The model under review builds one solid part; all positions refer to its coordinate system, in mm. A direction names the side the tool comes from. Round coordinates to 2 decimals unless told otherwise and drop trailing zeros. Write each loop counter-clockwise with the first axis right and the second up, starting at its lowest first coordinate (ties: lowest second). Pieces come first, ordered by that corner, then holes. Notation, with made-up numbers: (-38.75, 66.25) - (-31.75, 66.25) arc R27 cw to (-31.75, 87.25) - close; hole circle Ø1 at (11, 21). An arc over 180 degrees is marked (long way). Return JSON: item names as keys, results as strings.
from build123d import *

# Parameters (mm, degrees)
SKETCH_1_R          = 1.6
SKETCH_1_W          = 11.667697598
SKETCH_1_H          = 6.517356375
SKETCH_1_W_2        = 22
SKETCH_1_H_2        = 5
EXTRUDE_1_DEPTH     = 3
SKETCH_2_W          = 75.93825213
SKETCH_2_H          = 5.545458332
EXTRUDE_2_DEPTH     = 8
SKETCH_3_R          = 1.8
CUT_EXTRUDE_1_DEPTH = 15


with BuildPart() as part:
    # 草图1 → 凸台-拉伸1 (new body)
    with BuildSketch(Plane(origin=(0, 0, 0), x_dir=(1, 0, 0), z_dir=(0, 1, 0))):
        with BuildLine():
            Line((-49.5, -40), (49.5, -40))
            ThreePointArc((49.5, -40), (50.914213562, -39.414213562), (51.5, -38))
            Line((51.5, -38), (51.5, 38))
            ThreePointArc((51.5, 38), (50.914213562, 39.414213562), (49.5, 40))
            Line((49.5, 40), (20.187430173, 40))
            Line((20.187430173, 40), (20.187430173, 26.249140852))
            Line((20.187430173, 26.249140852), (-20.187430173, 26.249140852))
            Line((-20.187430173, 26.249140852), (-20.187430173, 40))
            Line((-20.187430173, 40), (-49.5, 40))
            ThreePointArc((-49.5, 40), (-50.914213562, 39.414213562), (-51.5, 38))
            Line((-51.5, 38), (-51.5, -38))
            ThreePointArc((-51.5, -38), (-50.914213562, -39.414213562), (-49.5, -40))
        make_face()
        with Locations(Location((-43.3, -31.8, 0), (0, 0, 270))):
            Circle(SKETCH_1_R, mode=Mode.SUBTRACT)
        with Locations((-30.135277266, -31.195863481)):
            Rectangle(SKETCH_1_W, SKETCH_1_H, mode=Mode.SUBTRACT)
        with Locations(Location((-42.391806281, -12.03, 0), (0, 0, 270))):
            Circle(SKETCH_1_R, mode=Mode.SUBTRACT)
        with Locations(Location((-33.901806281, -12.03, 0), (0, 0, 270))):
            Circle(SKETCH_1_R, mode=Mode.SUBTRACT)
        with Locations((0, -31.19586348)):
            Rectangle(SKETCH_1_W_2, SKETCH_1_H_2, mode=Mode.SUBTRACT)
        with Locations((30.135277266, -31.195863481)):
            Rectangle(SKETCH_1_W, SKETCH_1_H, mode=Mode.SUBTRACT)
        with Locations(Location((43.3, -31.8, 0), (0, 0, 270))):
            Circle(SKETCH_1_R, mode=Mode.SUBTRACT)
        with Locations(Location((33.901806281, -12.03, 0), (0, 0, 270))):
            Circle(SKETCH_1_R, mode=Mode.SUBTRACT)
        with Locations(Location((42.391806281, -12.03, 0), (0, 0, 270))):
            Circle(SKETCH_1_R, mode=Mode.SUBTRACT)
        with Locations(Location((-42.391806281, 12.03, 0), (0, 0, 270))):
            Circle(SKETCH_1_R, mode=Mode.SUBTRACT)
        with Locations(Location((-33.901806281, 12.03, 0), (0, 0, 270))):
            Circle(SKETCH_1_R, mode=Mode.SUBTRACT)
        with Locations(Location((-43.3, 31.8, 0), (0, 0, 270))):
            Circle(SKETCH_1_R, mode=Mode.SUBTRACT)
        with Locations(Location((33.901806281, 12.03, 0), (0, 0, 270))):
            Circle(SKETCH_1_R, mode=Mode.SUBTRACT)
        with Locations(Location((42.391806281, 12.03, 0), (0, 0, 270))):
            Circle(SKETCH_1_R, mode=Mode.SUBTRACT)
        with Locations(Location((43.3, 31.8, 0), (0, 0, 270))):
            Circle(SKETCH_1_R, mode=Mode.SUBTRACT)
    extrude(amount=EXTRUDE_1_DEPTH)

    # 草图2 → 凸台-拉伸2 (add)
    with BuildSketch(Plane(origin=(0, 3, 0), x_dir=(1, 0, 0), z_dir=(0, 1, 0))):
        with Locations((0, -37.227270834)):
            Rectangle(SKETCH_2_W, SKETCH_2_H)
    extrude(amount=-EXTRUDE_2_DEPTH)

    # 草图3 → 切除-拉伸1 (cut)
    with BuildSketch(Plane(origin=(0, -5, 0), x_dir=(-1, 0, 0), z_dir=(0, -1, 0))):
        with Locations(Location((30.875113943, -37.227270834, 0), (0, 0, 90))):
            Circle(SKETCH_3_R)
        with BuildLine():
            ThreePointArc((10, -37.227270834), (8.2, -35.427270834), (6.4, -37.227270834))
            Line((6.4, -37.227270834), (10, -37.227270834))
        make_face()
        with BuildLine():
            Line((10, -37.227270834), (6.4, -37.227270834))
            ThreePointArc((6.4, -37.227270834), (8.2, -39.027270834), (10, -37.227270834))
        make_face()
        with BuildLine():
            ThreePointArc((-10, -37.227270834), (-8.2, -39.027270834), (-6.4, -37.227270834))
            Line((-6.4, -37.227270834), (-10, -37.227270834))
        make_face()
        with BuildLine():
            Line((-10, -37.227270834), (-6.4, -37.227270834))
            ThreePointArc((-6.4, -37.227270834), (-8.2, -35.427270834), (-10, -37.227270834))
        make_face()
        with Locations(Location((-30.875113943, -37.227270834, 0), (0, 0, 90))):
            Circle(SKETCH_3_R)
    extrude(amount=-CUT_EXTRUDE_1_DEPTH, mode=Mode.SUBTRACT)


solid = part.part
(1) Mouldability with a two-part tool opening along Z and no side actions: class faces 1 (the flat face through (-35, 1, -40)), 2 (the flat face through (-35.969, 1, 31)), 3 (the flat face through (20.187, 1, -33)) as released by +Z, released by -Z, zero draft, split by the parting line, or undercut.
Filled in:
{"face 1": "released by -Z", "face 2": "undercut", "face 3": "zero draft"}
(2) Add section D-D (y = -2.25). Write out the cut boundary in (x, z).
Filled in:
{"outline": "(-37.97, 34.45) - (37.97, 34.45) - (37.97, 40) - (-37.97, 40) - close; hole circle Ø3.6 at (-30.88, 37.23); hole circle Ø3.6 at (-8.2, 37.23); hole circle Ø3.6 at (8.2, 37.23); hole circle Ø3.6 at (30.88, 37.23)"}
(3) Add section B-B (z = -31.8). Write out the cut boundary in (x, y).
Filled in:
{"outline": "(-51.5, 0) - (-44.9, 0) - (-44.9, 3) - (-51.5, 3) - close; (-41.7, 0) - (-20.19, 0) - (-20.19, 3) - (-41.7, 3) - close; (20.19, 0) - (41.7, 0) - (41.7, 3) - (20.19, 3) - close; (44.9, 0) - (51.5, 0) - (51.5, 3) - (44.9, 3) - close"}
(4) Clearance check with flat-ended pins moving along their axes: pin 1 Ø4 at (x, z) = (-42.39, -12.03) entering from -Y; pin 2 Ø2.5 at (x, y) = (7.5, -1) entering from -Z; pin 3 Ø2.5 at (y, z) = (-2, 37.5) entering from -X. State where each tip first meets the part, or that it passes through.
Filled in:
{"pin 1": "stops at y = 0", "pin 2": "stops at z = -26.25", "pin 3": "stops at x = -37.97"}
(5) For faces 4 (the flat face through (35.969, 1, 31)), 5 (the flat face through (0, 1, -26.249)), 6 (the cylindrical face through (-50.93, 1.48, 39.4)), list the 3-axis set-ups (+Z, -Z, +X, -X, +Y, -Y) from which the entire face can be reached by the end or side of a thin tool; tool diameter is ignored.
Filled in:
{"face 4": "+Y, -Y", "face 5": "-Z, +Y, -Y", "face 6": "+Z, -X, +Y, -Y"}
(6) Add section C-C (x = 8.2). Write out the cut boundary in (y, z).
Filled in:
{"outline": "(-5, 34.45) - (0, 34.45) - (0, 33.7) - (3, 33.7) - (3, 35.43) - (-5, 35.43) - close; (-5, 39.03) - (3, 39.03) - (3, 40) - (-5, 40) - close; (0, -26.25) - (3, -26.25) - (3, 28.7) - (0, 28.7) - close"}
(7) Wall thickness on line 1 (X direction, y = 0.7, z = -12.03); line 2 (X direction, y = 1.25, z = -34); line 3 (X direction, y = 2, z = -31.8): over which ranges is each line inside the solid? List them lowest first.
Filled in:
{"line 1": "x = -51.5 to -43.99, -40.79 to -35.5, -32.3 to 32.3, 35.5 to 40.79, 43.99 to 51.5", "line 2": "x = -51.5 to -20.19, 20.19 to 51.5", "line 3": "x = -51.5 to -44.9, -41.7 to -20.19, 20.19 to 41.7, 44.9 to 51.5"}
(8) Add section A-A (z = -12.03). Write out the cut boundary in (x, y).
Filled in:
{"outline": "(-51.5, 0) - (-43.99, 0) - (-43.99, 3) - (-51.5, 3) - close; (-40.79, 0) - (-35.5, 0) - (-35.5, 3) - (-40.79, 3) - close; (-32.3, 0) - (32.3, 0) - (32.3, 3) - (-32.3, 3) - close; (35.5, 0) - (40.79, 0) - (40.79, 3) - (35.5, 3) - close; (43.99, 0) - (51.5, 0) - (51.5, 3) - (43.99, 3) - close"}
